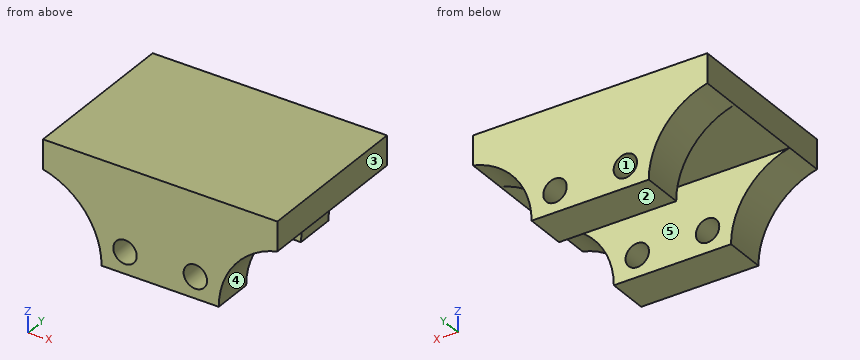
```python
from build123d import *

# Parameters (mm, degrees)
SKETCH2_W                = 400
SKETCH2_H                = 280
BOSS_EXTRUDE1_DEPTH      = 50
BOSS_EXTRUDE2_DEPTH      = 140
BOSS_EXTRUDE2_DEPTH_BACK = 140
CUT_EXTRUDE1_DEPTH       = 200
CUT_EXTRUDE1_DEPTH_BACK  = 200
SKETCH5_W                = 126.470213754
SKETCH5_H                = 140
CUT_EXTRUDE2_DEPTH       = 200
CUT_EXTRUDE2_DEPTH_BACK  = 200
SKETCH6_R                = 20


with BuildPart() as part:
    # Sketch2 → Boss-Extrude1 (new body)
    with BuildSketch(Plane.XY):
        Rectangle(SKETCH2_W, SKETCH2_H)
    extrude(amount=BOSS_EXTRUDE1_DEPTH)

    # Sketch4 → Boss-Extrude2 (add, two sides: drawn at the far end of the back side and taken through both)
    with BuildSketch(Plane(origin=(0, 0, 0), x_dir=(1, 0, 0), z_dir=(0, 1, 0)).offset(-BOSS_EXTRUDE2_DEPTH_BACK)):
        with BuildLine():
            Line((-100, 126.470213754), (100, 126.470213754))
            ThreePointArc((100, 126.470213754), (128.020392375, 45.855830783), (200, 0))
            Line((200, 0), (100, 0))
            Line((100, 0), (-100, 0))
            Line((-100, 0), (-200, 0))
            ThreePointArc((-200, 0), (-128.020392375, 45.855830783), (-100, 126.470213754))
        make_face()
    extrude(amount=BOSS_EXTRUDE2_DEPTH + BOSS_EXTRUDE2_DEPTH_BACK)

    # Sketch5 → Cut-Extrude1 (cut, two sides: drawn at the far end of the back side and taken through both)
    with BuildSketch(Plane(origin=(0, 0, 0), x_dir=(0, 0, -1), z_dir=(1, 0, 0)).offset(-CUT_EXTRUDE1_DEPTH_BACK)):
        with Locations((63.235106877, 0)):
            Rectangle(SKETCH5_W, SKETCH5_H)
    extrude(amount=CUT_EXTRUDE1_DEPTH + CUT_EXTRUDE1_DEPTH_BACK, mode=Mode.SUBTRACT)

    # Sketch6 → Cut-Extrude2 (cut, two sides: drawn at the far end of the back side and taken through both)
    with BuildSketch(Plane(origin=(0, 0, 0), x_dir=(1, 0, 0), z_dir=(0, 1, 0)).offset(-CUT_EXTRUDE2_DEPTH_BACK)):
        with Locations(Location((-60, 90, 0), (0, 0, 270))):
            Circle(SKETCH6_R)
        with Locations(Location((60, 90, 0), (0, 0, 270))):
            Circle(SKETCH6_R)
    extrude(amount=CUT_EXTRUDE2_DEPTH + CUT_EXTRUDE2_DEPTH_BACK, mode=Mode.SUBTRACT)


solid = part.part
```
Model file for the job. Use its own axes, mm. Face numbers are marked on the shaded views. A direction names the side the tool comes from. Coordinates: 2 decimals unless noted, no trailing zeros. Write each loop counter-clockwise with the first axis right and the second up, starting at its lowest first coordinate (ties: lowest second). Pieces come first, ordered by that corner, then holes. Notation, with made-up numbers: (56.5, -8.75) - (66.5, -8.75) arc R29 ccw to (66.5, 23.25) - close; hole circle Ø3 at (52, -36). An arc over 180 degrees is marked (long way). Use a Markdown table: item, result. Add a question column.
Item 1: Band-saw the part on B-B, the plane x = -60. Write the cut outline in (y, z).
Item 2: Band-saw the part on D-D, the plane x = -19. Write the cut outline in (y, z), and give its area (3 significant figures).
Item 3: Drop flat-ended pins along their axis: pin 1 (24 mm diameter, centred on x = -60, z = -90, fed in from -Y); pin 2 (2 mm diameter, centred on x = 89.5, y = -17, fed in from -Z). Give the stop position or say it passes through.
Item 4: 3-axis set-ups, long thin cutter, end or side, ignore diameter. For the marked faces 4 and 5: which of +Z, -Z, +X, -X, +Y, -Y reach the whole face in a straight line?
Item 5: Drill centre lines: line 1 along Z through (x, y) = (60, 100); line 2 along X through (y, z) = (84, -90); line 3 along Y through (x, z) = (100, -39.5). Where is each one in solid material? Low to high.
Item 6: Band-saw the part on A-A, the plane y = -102. Write the cut outline in (x, z), and give its area (3 significant figures).
Item 7: Band-saw the part on C-C, the plane z = -87. Write the cut outline in (x, y), and give its area (3 significant figures).
Item 8: Two-plate mould, pull along Z, no slides. Class the marked faces 1, 2 and 3: pulls with the +Z half, pulls with the -Z half, needs draft (parallel to the pull), parting line crosses it, or undercut.
A:
| question | item | result |
|---|---|---|
| 1 | outline | (-140, -126.47) - (-70, -126.47) - (-70, -110) - (-140, -110) - close; (-140, -70) - (-70, -70) - (-70, 0) - (70, 0) - (70, -70) - (140, -70) - (140, 50) - (-140, 50) - close; (70, -126.47) - (140, -126.47) - (140, -110) - (70, -110) - close |
| 2 | outline | (-140, -126.47) - (-70, -126.47) - (-70, 0) - (70, 0) - (70, -126.47) - (140, -126.47) - (140, 50) - (-140, 50) - close |
| 2 | area | 31,700 mm² |
| 3 | pin 1 | passes through |
| 3 | pin 2 | stops at z = 0 |
| 4 | face 4 | -Z, +X, +Y, -Y |
| 4 | face 5 | -Z, +X, -X |
| 5 | line 1 | z = -126.47 to -110, -70 to 50 |
| 5 | line 2 | x = -105.22 to -80, -40 to 40, 80 to 105.22 |
| 5 | line 3 | y = -140 to -70, 70 to 140 |
| 6 | outline | (-200, 0) arc R129.97 cw to (-100, -126.47) - (100, -126.47) arc R129.97 cw to (200, 0) - (200, 50) - (-200, 50) - close; hole circle Ø40 at (-60, -90); hole circle Ø40 at (60, -90) |
| 6 | area | 49,300 mm² |
| 7 | outline | (-106.14, -140) - (-79.77, -140) - (-79.77, -70) - (-106.14, -70) - close; (-106.14, 70) - (-79.77, 70) - (-79.77, 140) - (-106.14, 140) - close; (-40.23, -140) - (40.23, -140) - (40.23, -70) - (-40.23, -70) - close; (-40.23, 70) - (40.23, 70) - (40.23, 140) - (-40.23, 140) - close; (79.77, -140) - (106.14, -140) - (106.14, -70) - (79.77, -70) - close; (79.77, 70) - (106.14, 70) - (106.14, 140) - (79.77, 140) - close |
| 7 | area | 18,600 mm² |
| 8 | face 1 | undercut |
| 8 | face 2 | pulls with the -Z half |
| 8 | face 3 | needs draft |
